from build123d import *

# Parameters (mm, degrees)
SKETCH2_W                = 268
SKETCH2_H                = 172.5
BOSS_EXTRUDE2_DEPTH      = 5.2
BOSS_EXTRUDE1_DEPTH      = 6.2
BOSS_EXTRUDE1_DEPTH_BACK = 33
SKETCH1_W                = 244
SKETCH1_H                = 148.4
M4_CLEARANCE_HOLE1_D     = 4.5
SKETCH6_W                = 149.557953786
SKETCH6_H                = 93.729813504
CUT_EXTRUDE1_DEPTH       = 1
SKETCH7_W                = 10.202720683
SKETCH7_H                = 115.902906959
SKETCH7_W_2              = 155.285408795
SKETCH7_H_2              = 10.202720683
SKETCH7_W_3              = 157.734061759
SKETCH7_H_3              = 10.61082951
BOSS_EXTRUDE3_DEPTH      = 10


with BuildPart() as part:
    # Sketch2 → Boss-Extrude2 (new body)
    with BuildSketch(Plane.XY):
        Rectangle(SKETCH2_W, SKETCH2_H)
    extrude(amount=BOSS_EXTRUDE2_DEPTH)

    # Sketch1 → Boss-Extrude1 (add, two sides: drawn at the far end of the back side and taken through both)
    with BuildSketch(Plane.XY.offset(-BOSS_EXTRUDE1_DEPTH_BACK)):
        Rectangle(SKETCH1_W, SKETCH1_H)
    extrude(amount=BOSS_EXTRUDE1_DEPTH + BOSS_EXTRUDE1_DEPTH_BACK)

    # M4 Clearance Hole1 (through all)
    with Locations(Plane(origin=(0, 0, 0), x_dir=(-1, 0, 0), z_dir=(0, 0, -1))):
        with Locations((-129.2, 54.5), (129.2, -54.5), (129.2, 54.5), (-129.2, -54.5)):
            Hole(M4_CLEARANCE_HOLE1_D / 2)

    # Sketch6 → Cut-Extrude1 (cut)
    with BuildSketch(Plane.XY.offset(6.2)):
        with Locations((-32.438368972, 16.987461646)):
            Rectangle(SKETCH6_W, SKETCH6_H)
    extrude(amount=-CUT_EXTRUDE1_DEPTH, mode=Mode.SUBTRACT)

    # Sketch7 → Boss-Extrude3 (add)
    with BuildSketch(Plane(origin=(0, 0, -33), x_dir=(-1, 0, 0), z_dir=(0, 0, -1))):
        with Locations((-98.57020546, 0.991507772)):
            Rectangle(SKETCH7_W, SKETCH7_H)
        with Locations((0.090103545, 59.555124492)):
            Rectangle(SKETCH7_W_2, SKETCH7_H_2)
        with Locations((4.579300645, -53.899129503)):
            Rectangle(SKETCH7_W_3, SKETCH7_H_3)
    extrude(amount=BOSS_EXTRUDE3_DEPTH)


solid = part.part
Design review of the part built by this model. Coordinates are the model's own, in mm. A direction names the side the tool comes from. Give positions to 0.01 mm unless a question says otherwise; leave off trailing zeros. Write each loop counter-clockwise with the first axis right and the second up, starting at its lowest first coordinate (ties: lowest second). Pieces come first, ordered by that corner, then holes. Notation, with made-up numbers: M 67.5,-9 L 102.5,-9 A24 cw 102.5,29 Z; hole C 10.25,-13 d1. An arc over 180 degrees is marked long. Answer as a JSON object with one key per item and string values. Group by question number.
1) We need section B-B (x = 110.5). Give the boundary of the cut face in (y, z), and give its area (3 significant figures).
2) We need section A-A (z = -38.5). Give the boundary of the cut face in (x, y).
3) Mouldability with a two-part tool opening along Y and no side actions: class faces 1 (the face through (-2, 1, -33)), 2 (the face through (-2, -74.2, -17)), 3 (the face through (1, 64.656, -38)), 4 (the face through (134, -1, 3)) as released by +Y, released by -Y, zero draft, split by the parting line, or undercut.
4) We need section C-C (y = -17.5). Give the boundary of the cut face in (x, z).
5) For line 1 along Y through (x, z) = (-129.2, 3.85); line 2 along X through (y, z) = (-54, 2); line 3 along Y through (x, z) = (61.5, -38), list the stretches that pass through material, from the lowest coordinate up.
6) Clearance check with flat-ended pins moving along their axes: pin 1 Ø0.8 at (x, z) = (-54.5, 6) entering from +Y; pin 2 Ø5 at (x, z) = (8.5, -36) entering from +Y; pin 3 Ø8 at (y, z) = (-54, -39.5) entering from -X. State where each tip first meets the part, or that it passes through.
7) We need section D-D (y = 70.5). Give the boundary of the cut face in (x, z).
8) Tool access review of faces 5 (the face through (-77.733, 59, -38)), 6 (the face through (-3, -59.205, -38)), 7 (the face through (-3, -48.594, -38)), 8 (the face through (-2, 74.2, -17)): name each direction out of +Z, -Z, +X, -X, +Y, -Y from which nothing blocks a thin tool from reaching the whole face with its end or side.
Answer key:
{
 "1": {"outline": "M -86.25,0 L -74.2,0 L -74.2,-33 L 74.2,-33 L 74.2,0 L 86.25,0 L 86.25,5.2 L 74.2,5.2 L 74.2,6.2 L -74.2,6.2 L -74.2,5.2 L -86.25,5.2 Z", "area": "5,940 mm²"},
 "2": {"outline": "M -83.45,-59.2 L 74.29,-59.2 L 74.29,-48.59 L -83.45,-48.59 Z; M -77.73,54.45 L 77.55,54.45 L 77.55,64.66 L -77.73,64.66 Z; M 93.47,-56.96 L 103.67,-56.96 L 103.67,58.94 L 93.47,58.94 Z"},
 "3": {"face 1": "undercut", "face 2": "released by -Y", "face 3": "released by +Y", "face 4": "zero draft"},
 "4": {"outline": "M -134,0 L -122,0 L -122,-33 L 93.47,-33 L 93.47,-43 L 103.67,-43 L 103.67,-33 L 122,-33 L 122,0 L 134,0 L 134,5.2 L 122,5.2 L 122,6.2 L 42.34,6.2 L 42.34,5.2 L -107.22,5.2 L -107.22,6.2 L -122,6.2 L -122,5.2 L -134,5.2 Z"},
 "5": {"line 1": "y = -86.25 to -56.75, -52.25 to 52.25, 56.75 to 86.25", "line 2": "x = -134 to -131.39, -127.01 to 127.01, 131.39 to 134", "line 3": "y = -59.2 to -48.59, 54.45 to 64.66"},
 "6": {"pin 1": "stops at y = 74.2", "pin 2": "stops at y = 64.66", "pin 3": "stops at x = -83.45"},
 "7": {"outline": "M -134,0 L -122,0 L -122,-33 L 122,-33 L 122,0 L 134,0 L 134,5.2 L 122,5.2 L 122,6.2 L -122,6.2 L -122,5.2 L -134,5.2 Z"},
 "8": {"face 5": "-Z, -X, +Y", "face 6": "-Z, +X, -X, -Y", "face 7": "-Z, -X", "face 8": "-Z, +X, -X, +Y"}
}
